Autodesk Inventor part; units mm, degrees
ref_plane "YZ Plane" through (0, 0, 0) normal (1, 0, 0) x (0, 1, 0)
ref_plane "XZ Plane" through (0, 0, 0) normal (0, 1, 0) x (-1, 0, 0)
ref_plane "XY Plane" through (0, 0, 0) normal (0, 0, 1) x (1, 0, 0)
sketch "Эскиз1" plane through (0, 0, 0) normal (0, 0, 1) x (1, 0, 0)
  line L0 (10.4, -8.25) -> (-10.4, -8.25)
  line L1 (-10.4, -8.25) -> (-10.4, 8.25)
  line L2 (-10.4, 8.25) -> (10.4, 8.25)
  line L3 (10.4, 8.25) -> (10.4, -8.25)
  line L4 (10.4, -8.25) -> (-10.4, 8.25) construction
  line L5 (-10.4, -8.25) -> (10.4, 8.25) construction
  circle A0 centre (-8.25, -6.25) radius 1.5
  circle A1 centre (8.25, -6.25) radius 1.5
  circle A2 centre (-9.1, 6.95) radius 0.5
  circle A3 centre (-9.1, 6.95) radius 0.875
  line L6 (-10.4, 6.95) -> (10.4, 6.95) construction
  point P0 (0, 0)
  dimension "d0" = 20.8
  dimension "d1" = 16.5
  dimension "d2" = 3
  dimension "d3" = 3
  dimension "d4" = 13.5
  dimension "d5" = 0.5
  dimension "d8" = 2.15
  dimension "d9" = 2.15
  dimension "d10" = 1
  dimension "d11" = 1.75
  dimension "d12" = 1.3
  dimension "d13" = 1.3
extrude "Выдавливание1" add sketch "Эскиз1" along normal blind 1 contours L0 L1 L2 L3 | A2 | A3
extrude "Выдавливание2" cut sketch "Эскиз1" along normal blind 1.5 contours A2
extrude "Выдавливание3" add sketch "Эскиз1" along normal blind 0.1 from surface at 1 contours A3
pattern_linear "Прямоуг.массив1" count 8 spacing 2.6 along (1, 0, 0) of "Выдавливание3", "Выдавливание2"
sketch "Эскиз2" plane through (0, 0, 1) normal (0, 0, 1) x (1, 0, 0)
  line L0 (2.3179, -3.0275) -> (-2.1648, -3.0275)
  line L1 (-2.1648, -3.0275) -> (-2.1648, 1.3166)
  line L2 (-2.1648, 1.3166) -> (2.3179, 1.3166)
  line L3 (2.3179, 1.3166) -> (2.3179, -3.0275)
  line L4 (2.3179, -3.0275) -> (-2.1648, 1.3166) construction
  line L5 (-2.1648, -3.0275) -> (2.3179, 1.3166) construction
  line L6 (-2.1648, -5.8271) -> (2.1648, -5.8271)
  line L7 (2.1648, -5.8271) -> (2.1648, -7.3246)
  line L8 (2.1648, -7.3246) -> (-2.1648, -7.3246)
  line L9 (-2.1648, -7.3246) -> (-2.1648, -5.8271)
  line L10 (-2.1648, -5.8271) -> (2.1648, -7.3246) construction
  line L11 (2.1648, -5.8271) -> (-2.1648, -7.3246) construction
  line L12 (-7.6013, 2.4415) -> (-6.82, 2.4415)
  line L13 (-6.82, 2.4415) -> (-6.82, 1.0092)
  line L14 (-6.82, 1.0092) -> (-7.6013, 1.0092)
  line L15 (-7.6013, 1.0092) -> (-7.6013, 2.4415)
  line L16 (-7.6013, 2.4415) -> (-6.82, 1.0092) construction
  line L17 (-6.82, 2.4415) -> (-7.6013, 1.0092) construction
  line L18 (4.8419, 3.8739) -> (6.1364, 3.8739)
  line L19 (6.1364, 3.8739) -> (6.1364, 1.0092)
  line L20 (6.1364, 1.0092) -> (4.8419, 1.0092)
  line L21 (4.8419, 1.0092) -> (4.8419, 3.8739)
  line L22 (4.8419, 3.8739) -> (6.1364, 1.0092) construction
  line L23 (6.1364, 3.8739) -> (4.8419, 1.0092) construction
  line L24 (-3.7552, 4.3914) -> (-1.058, 4.3914)
  line L25 (-1.058, 4.3914) -> (-1.058, 2.4415)
  line L26 (-1.058, 2.4415) -> (-3.7552, 2.4415)
  line L27 (-3.7552, 2.4415) -> (-3.7552, 4.3914)
  line L28 (-3.7552, 4.3914) -> (-1.058, 2.4415) construction
  line L29 (-1.058, 4.3914) -> (-3.7552, 2.4415) construction
  line L30 (-7.6406, -1.8556) -> (-5.153, -1.8556)
  line L31 (-5.153, -1.8556) -> (-5.153, -3.2228)
  line L32 (-5.153, -3.2228) -> (-7.6406, -3.2228)
  line L33 (-7.6406, -3.2228) -> (-7.6406, -1.8556)
  line L34 (-7.6406, -1.8556) -> (-5.153, -3.2228) construction
  line L35 (-5.153, -1.8556) -> (-7.6406, -3.2228) construction
  point P0 (0, 0)
  point P1 (0.0765, -0.8555)
  point P2 (0, -6.5758)
  point P3 (-7.2106, 1.7253)
  point P4 (5.4892, 2.4415)
  point P5 (-2.4066, 3.4165)
  point P6 (-6.3968, -2.5392)
extrude "Выдавливание4" add sketch "Эскиз2" along normal blind 0.3 contours L0 L1 L2 L3
extrude "Выдавливание5" add sketch "Эскиз2" along normal blind 1.5 contours L6 L7 L8 L9
extrude "Выдавливание6" add sketch "Эскиз2" along normal blind 0.5 contours L12 L13 L14 L15 | L18 L19 L20 L21 | L24 L25 L26 L27 | L30 L31 L32 L33
sketch "Эскиз3" plane through (0, 0, 1.3) normal (0, 0, 1) x (1, 0, 0)
  line L0 (2.3179, 1.3166) -> (-2.1648, 1.3166) construction
  line L1 (-2.1648, 1.3166) -> (-2.1648, -3.0275) construction
  line L2 (-2.1648, -3.0275) -> (2.3179, -3.0275) construction
  line L3 (2.3179, -3.0275) -> (2.3179, 1.3166) construction
  point P0 (0, 0)
  point P1 (0.0765, -0.8555)
  point P2 (0.0765, 1.3166)
  point P3 (2.3179, -0.8555)
equation "\"d8\" = d9"
equation "\"d13\" = 0.0625 * d0"
equation "\"d22\" = 2 * d13"
properties part number "MPU6050"
The model under review builds one solid part; all positions refer to its coordinate system, in mm. A direction names the side the tool comes from. Round coordinates to 2 decimals unless told otherwise and drop trailing zeros. Loops run counter-clockwise (first coordinate to the right, second up) from the corner with the lowest first, then second, coordinate; pieces in that order, holes last. Notation, with made-up numbers: (-38.75, -6.75) -> (13.25, -6.75) arc R17 cw to (13.25, 3.25) -> close; hole circle Ø11 at (25.25, -22.75). An arc over 180 degrees is marked (long way). Write item = value, one per line. Start each with the question number.
Item 1: Take a section at A-A on x = 3.9. Give the boundary of the cut face in (y, z) (3 decimals), plus the area to 3 significant figures.
Item 2: For faces 1 (the flat face through (0, -7.325, 2)), 2 (the flat face through (0, -7, 2.5)), 3 (the flat face through (0, -5.827, 2)), list the 3-axis set-ups (+Z, -Z, +X, -X, +Y, -Y) from which the entire face can be reached by the end or side of a thin tool; tool diameter is ignored.
Item 3: Take a section at D-D on x = -2.75. Give the boundary of the cut face in (y, z).
Item 4: Insertion check: pin 1 (1.3 mm diameter, centred on x = -0.5, y = -0.5, fed in from +Z); pin 2 (4 mm diameter, centred on x = 0, y = 2, fed in from +Z); pin 3 (1.5 mm diameter, centred on y = 2, z = 1.5, fed in from -X); pin 4 (0.5 mm diameter, centred on x = -3.5, y = 6.5, fed in from +Z). Each pin has a flat end and moves straight along its axis. Give the tip position at first contact, or say it passes through.
Item 5: Mouldability with a two-part tool opening along Y and no side actions: class faces 4 (the cylindrical face through (-9.75, -6.32, 0.49)), 5 (the flat face through (-0.1, 8.25, 0.5)), 6 (the flat face through (10.4, 0.1, 0.5)) as released by +Y, released by -Y, zero draft, split by the parting line, or undercut.
Item 6: Take a section at C-C on y = -1.25. Give the boundary of the cut face in (x, z), plus the area to 3 significant figures.
Item 7: To check wall thickness, follow L1, parallel to Y at x = 1.25, z = 0.7; L2, parallel to Y at x = 9.1, z = 0.3; L3, parallel to Z at x = 6, y = -0.75. State the ranges of each line that lie inside material, in increasing order.
Item 8: Take a section at B-B on z = 0.35. Count the separate pieces of the cut face and the enclosed holes in it, plus the area to 3 significant figures.
Result:
q1.outline = (-8.25, 0) -> (6.45, 0) -> (6.45, 1.1) -> (6.075, 1.1) -> (6.075, 1) -> (-8.25, 1) -> close; (7.45, 0) -> (8.25, 0) -> (8.25, 1) -> (7.825, 1) -> (7.825, 1.1) -> (7.45, 1.1) -> close
q1.area = 15.6 mm²
q2.face_1 = +Z, +X, -X, -Y
q2.face_2 = +Z, +X, -X, +Y, -Y
q2.face_3 = +Z, +X, -X
q3.outline = (-8.25, 0) -> (8.25, 0) -> (8.25, 1) -> (4.39, 1) -> (4.39, 1.5) -> (2.44, 1.5) -> (2.44, 1) -> (-8.25, 1) -> close
q4.pin_1 = 1.3
q4.pin_2 = 1.5
q4.pin_3 = -10.4
q4.pin_4 = 1.1
q5.face_4 = undercut
q5.face_5 = released by +Y
q5.face_6 = zero draft
q6.outline = (-10.4, 0) -> (10.4, 0) -> (10.4, 1) -> (2.32, 1) -> (2.32, 1.3) -> (-2.16, 1.3) -> (-2.16, 1) -> (-10.4, 1) -> close
q6.area = 22.1 mm²
q7.L1 = -8.25 to 6.45, 7.45 to 8.25
q7.L2 = -8.25 to -7.49, -5.01 to 6.45, 7.45 to 8.25
q7.L3 = 0 to 1
q8.separate_pieces = 1
q8.enclosed_holes = 10
q8.area = 323 mm²
